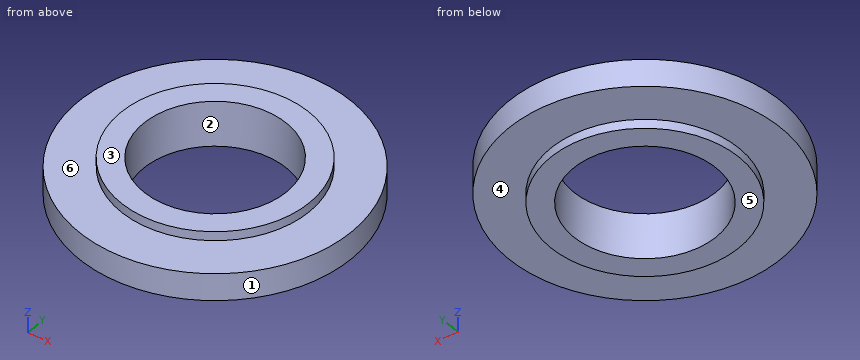
from build123d import *

# Parameters (mm, degrees)
SKETCH_1_R          = 6
SKETCH_1_R_2        = 3.15
EXTRUDE_1_DEPTH     = 2
CUT_EXTRUDE_START   = -0.4
SKETCH_2_R          = 6
SKETCH_2_R_2        = 4.15
CUT_EXTRUDE_1_DEPTH = 0.4
CUT_EXTRUDE_START_2 = -2
SKETCH_2_2_R        = 6
SKETCH_2_2_R_2      = 4.15
CUT_EXTRUDE_2_DEPTH = 0.4


with BuildPart() as part:
    # ｽｹｯﾁ1 → ﾎﾞｽ - 押し出し1 (new body)
    with BuildSketch(Plane.XY):
        Circle(SKETCH_1_R)
        Circle(SKETCH_1_R_2, mode=Mode.SUBTRACT)
    extrude(amount=EXTRUDE_1_DEPTH)

    # ｽｹｯﾁ2 → ｶｯﾄ - 押し出し1 (cut)
    with BuildSketch(Plane.XY.offset(2).offset(CUT_EXTRUDE_START)):
        Circle(SKETCH_2_R)
        Circle(SKETCH_2_R_2, mode=Mode.SUBTRACT)
    extrude(amount=CUT_EXTRUDE_1_DEPTH, mode=Mode.SUBTRACT)

    # ｽｹｯﾁ2<2> → ｶｯﾄ - 押し出し2 (cut)
    with BuildSketch(Plane.XY.offset(2).offset(CUT_EXTRUDE_START_2)):
        Circle(SKETCH_2_2_R)
        Circle(SKETCH_2_2_R_2, mode=Mode.SUBTRACT)
    extrude(amount=CUT_EXTRUDE_2_DEPTH, mode=Mode.SUBTRACT)


solid = part.part
Check sheet for the modelled part. Datum: model origin and axes. Units: mm. Face numbers are marked on the shaded views. A direction names the side the tool comes from. Round coordinates to 2 decimals unless told otherwise and drop trailing zeros. Loops run counter-clockwise (first coordinate to the right, second up) from the corner with the lowest first, then second, coordinate; pieces in that order, holes last.
1. Scan lines: probe 1 along Y at (x, z) = (0, 0.95); probe 2 along Y at (x, z) = (0, 1.85); probe 3 along Z at (x, y) = (2.5, 3.5). Record each from-to range of solid material in increasing order.
2. Gauge pin test, flat end, axial feed: pin 1 Ø7 at (x, y) = (0, 0) entering from -Z. Record the tip position at first contact, or that the pin passes through.
3. Sectioned sample at A-A on x = 0. Record the boundary of the cut face in (y, z).
4. Set-up check for the marked faces 4, 5 and 6: record each of +Z, -Z, +X, -X, +Y, -Y from which the full face is reachable in a straight line by a thin tool's end or side.
5. Mould release check, pull along Y, two halves, no side actions. Record for the marked faces 1, 2 and 3: released by +Y, released by -Y, zero draft, split by the parting line, or undercut.
6. Sectioned sample at D-D on x = 3.75. Record the boundary of the cut face in (y, z).
7. Sectioned sample at C-C on z = 0.25. Record the boundary of the cut face in (x, y).
Recorded:
1. probe 1: y = -6 to -3.15, 3.15 to 6
1. probe 2: y = -4.15 to -3.15, 3.15 to 4.15
1. probe 3: z = 0.4 to 1.6
2. pin 1: stops at z = 0
3. outline: (-6, 0.4) - (-4.15, 0.4) - (-4.15, 0) - (-3.15, 0) - (-3.15, 2) - (-4.15, 2) - (-4.15, 1.6) - (-6, 1.6) - close; (3.15, 0) - (4.15, 0) - (4.15, 0.4) - (6, 0.4) - (6, 1.6) - (4.15, 1.6) - (4.15, 2) - (3.15, 2) - close
4. face 4: -Z
4. face 5: -Z, +X, -X, +Y, -Y
4. face 6: +Z
5. face 1: split by the parting line
5. face 2: undercut
5. face 3: zero draft
6. outline: (-4.68, 0.4) - (-1.78, 0.4) - (-1.78, 0) - (1.78, 0) - (1.78, 0.4) - (4.68, 0.4) - (4.68, 1.6) - (1.78, 1.6) - (1.78, 2) - (-1.78, 2) - (-1.78, 1.6) - (-4.68, 1.6) - close
7. outline: circle Ø8.3 at (0, 0); hole circle Ø6.3 at (0, 0)
